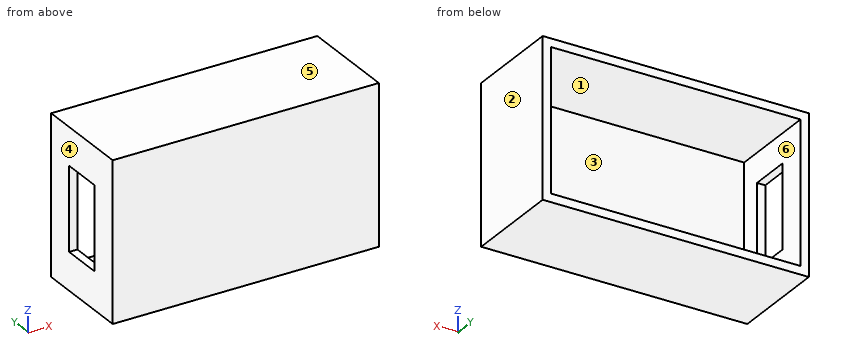
from build123d import *

# Parameters (mm, degrees)
CROQUIS1_W              = 32
CROQUIS1_H              = 19
CROQUIS1_W_2            = 30
CROQUIS1_H_2            = 17
SALIENTE_EXTRUIR1_DEPTH = 12
CROQUIS1_3_W            = 30
CROQUIS1_3_H            = 17
SALIENTE_EXTRUIR2_DEPTH = 1
CROQUIS2_W              = 5
CROQUIS2_H              = 5
CORTAR_EXTRUIR1_DEPTH   = 1


with BuildPart() as part:
    # Croquis1 → Saliente-Extruir1 (new body)
    with BuildSketch(Plane(origin=(0, 0, 0), x_dir=(1, 0, 0), z_dir=(0, 1, 0))):
        with Locations((15, 8.5)):
            Rectangle(CROQUIS1_W, CROQUIS1_H)
        with Locations((15, 8.5)):
            Rectangle(CROQUIS1_W_2, CROQUIS1_H_2, mode=Mode.SUBTRACT)
    extrude(amount=SALIENTE_EXTRUIR1_DEPTH)

    # Croquis1_3 → Saliente-Extruir2 (add)
    with BuildSketch(Plane(origin=(0, 0, 0), x_dir=(1, 0, 0), z_dir=(0, 1, 0))):
        with Locations((15, 8.5)):
            Rectangle(CROQUIS1_3_W, CROQUIS1_3_H)
    extrude(amount=SALIENTE_EXTRUIR2_DEPTH)

    # Croquis2 → Cortar-Extruir1 (cut)
    with BuildSketch(Plane.ZY.offset(1)):
        with Locations((-11, 6)):
            Rectangle(CROQUIS2_W, CROQUIS2_H)
        with Locations((-6, 6)):
            Rectangle(CROQUIS2_W, CROQUIS2_H)
    extrude(amount=-CORTAR_EXTRUIR1_DEPTH, mode=Mode.SUBTRACT)


solid = part.part
Verification items for the finished model (mm, model axes). Face numbers are marked on the shaded views. A direction names the side the tool comes from. Round coordinates to 2 decimals unless told otherwise and drop trailing zeros. Loops run counter-clockwise (first coordinate to the right, second up) from the corner with the lowest first, then second, coordinate; pieces in that order, holes last. Notation, with made-up numbers: M 38.25,12 L 96.25,12 A23 cw 96.25,21 Z; hole C 26.5,-20.5 d6. An arc over 180 degrees is marked long. Write each question's results on one line, items separated by ' | '.
1) Gauge pin test, flat end, axial feed: P1, Ø5, axis at x = 9.5, z = -8.5, coming from the +Y side. Record the tip position at first contact, or that the pin passes through.
Checks:
P1: stops at y = 1
2) Access from +Z, -Z, +X, -X, +Y, -Y to the whole of each face (thin tool, end or side, straight path). Record for the marked faces 1 and 2.
Checks:
face 1: +Y | face 2: +Z, -Z, +X, +Y, -Y
3) Section check D-D on y = 6.5. Record the boundary of the cut face in (x, z).
Checks:
outline: M -1,-18 L 31,-18 L 31,1 L -1,1 L -1,-3.5 L 0,-3.5 L 0,0 L 30,0 L 30,-17 L 0,-17 L 0,-13.5 L -1,-13.5 Z
4) Section check A-A on y = 2. Record the boundary of the cut face in (x, z).
Checks:
outline: M -1,-18 L 31,-18 L 31,1 L -1,1 Z; hole M 0,-17 L 30,-17 L 30,0 L 0,0 Z
5) Mould release check, pull along X, two halves, no side actions. Record for the marked faces 3, 4, 5 and 6: released by +X, released by -X, zero draft, split by the parting line, or undercut.
Checks:
face 3: undercut | face 4: released by -X | face 5: zero draft | face 6: undercut
6) Section check B-B on z = -4.5. Record the boundary of the cut face in (x, y), then the cut area to 3 significant figures.
Checks:
outline: M -1,0 L 31,0 L 31,12 L 30,12 L 30,1 L 0,1 L 0,3.5 L -1,3.5 Z; M -1,8.5 L 0,8.5 L 0,12 L -1,12 Z | area: 49.0 mm2
7) Section check C-C on x = 17.5. Record the boundary of the cut face in (y, z).
Checks:
outline: M 0,-18 L 12,-18 L 12,-17 L 1,-17 L 1,0 L 12,0 L 12,1 L 0,1 Z
8) Scan lines: L1, parallel to X at y = 1.5, z = -10.75; L2, parallel to Z at x = 25.5, y = 2.5; L3, parallel to X at y = 6.5, z = -11. Record each from-to range of solid material in increasing order. Write a range as from..to.
Checks:
L1: x = -1..0, 30..31 | L2: z = -18..-17, 0..1 | L3: x = 30..31
